from build123d import *

# Parameters (mm, degrees)
SKETCH2_W               = 147.5
SKETCH2_H               = 176.75
BOSS_EXTRUDE1_DEPTH     = 10
SKETCH3_W               = 29
SKETCH3_H               = 15
BOSS_EXTRUDE2_DEPTH     = 34
BOSS_EXTRUDE3_DEPTH     = 34
SKETCH8_W               = 113.5
SKETCH8_H               = 176.75
CUT_EXTRUDE1_DEPTH      = 30
SKETCH9_R               = 2.5
CUT_EXTRUDE2_DEPTH      = 134.016415209
SKETCH10_W              = 3
SKETCH10_H              = 3
CUT_EXTRUDE3_DEPTH      = 3
CUT_EXTRUDE4_DEPTH      = 134.016415209
CUT_EXTRUDE4_DEPTH_BACK = 134.016415209
SKETCH11_W              = 9
SKETCH11_H              = 8
SKETCH11_H_2            = 4
SKETCH11_W_2            = 3
SKETCH11_R              = 2.5
SKETCH11_W_3            = 34
SKETCH11_H_3            = 15
CUT_EXTRUDE5_DEPTH      = 94.691731892
CUT_EXTRUDE5_DEPTH_BACK = 94.691731892
SKETCH13_R              = 2.5
CUT_EXTRUDE6_DEPTH      = 94.691731892
CUT_EXTRUDE6_DEPTH_BACK = 94.691731892
SKETCH14_W              = 10
SKETCH14_H              = 2
FILLET1_R               = 2
SKETCH15_R              = 1.4
CUT_EXTRUDE7_DEPTH      = 34
SKETCH18_W              = 12
SKETCH18_H              = 8
CUT_EXTRUDE8_DEPTH      = 34
SKETCH19_W              = 7
SKETCH19_H              = 8
SKETCH19_W_2            = 12
CUT_EXTRUDE9_DEPTH      = 34
BOSS_EXTRUDE4_START     = 5
SKETCH20_W              = 34
SKETCH20_H              = 29
SKETCH20_R              = 1.4
BOSS_EXTRUDE4_DEPTH     = 5
SKETCH21_W              = 34
SKETCH21_H              = 29
SKETCH21_W_2            = 10
SKETCH21_H_2            = 10
CUT_EXTRUDE10_DEPTH     = 5
SKETCH22_W              = 10
SKETCH22_H              = 3
CUT_EXTRUDE11_DEPTH     = 1


with BuildPart() as part:
    # Sketch2 → Boss-Extrude1 (new body)
    with BuildSketch(Plane.XY):
        Rectangle(SKETCH2_W, SKETCH2_H)
    extrude(amount=BOSS_EXTRUDE1_DEPTH)

    # Sketch3 → Boss-Extrude2 (add)
    with BuildSketch(Plane.ZY.offset(73.75)):
        with Locations((7.5, 80.875)):
            Rectangle(SKETCH3_W, SKETCH3_H)
        with Locations((7.5, -80.875)):
            Rectangle(SKETCH3_W, SKETCH3_H)
    boss_extrude2 = extrude(amount=-BOSS_EXTRUDE2_DEPTH)

    # Mirror1: Boss-Extrude2 across plane
    add(boss_extrude2.mirror(Plane(origin=(0, 0, 0), x_dir=(0, 0, 1), z_dir=(1, 0, 0))))

    # Sketch5 → Boss-Extrude3 (add)
    with BuildSketch(Plane.ZY.offset(73.75)):
        Polygon((13.717233978, 0), (47.494362324, 23.650999887), (54.37727956, 13.821175356), (66.664560225, 22.424821901), (50.030843571, 46.180231185), (37.743562906, 37.57658464), (41.758597961, 31.84252033), (10, 9.604910635), (10, -9.604910635), (41.758597961, -31.84252033), (37.743562906, -37.57658464), (50.030843571, -46.180231185), (66.664560225, -22.424821901), (54.37727956, -13.821175356), (47.494362324, -23.650999887), align=None)
    extrude(amount=-BOSS_EXTRUDE3_DEPTH)

    # Sketch8 → Cut-Extrude1 (cut)
    with BuildSketch(Plane.XY.offset(22)):
        with Locations((17, 0)):
            Rectangle(SKETCH8_W, SKETCH8_H)
    extrude(amount=-CUT_EXTRUDE1_DEPTH, mode=Mode.SUBTRACT)

    # Sketch9 → Cut-Extrude2 (cut, through all)
    with BuildSketch(Plane(origin=(0, 0, 0), x_dir=(-1, 0, 0), z_dir=(0, 0, -1))):
        with Locations((49.75, 58.375)):
            Circle(SKETCH9_R)
        with Locations((63.75, 58.375)):
            Circle(SKETCH9_R)
        with Locations((49.75, -53.375)):
            Circle(SKETCH9_R)
        with Locations((63.75, -53.375)):
            Circle(SKETCH9_R)
    extrude(amount=-CUT_EXTRUDE2_DEPTH, mode=Mode.SUBTRACT)

    # Sketch10 → Cut-Extrude3 (cut)
    with BuildSketch(Plane(origin=(0, 0, -7), x_dir=(-1, 0, 0), z_dir=(0, 0, -1))):
        with Locations((72.25, 86.875)):
            Rectangle(SKETCH10_W, SKETCH10_H)
    extrude(amount=-CUT_EXTRUDE3_DEPTH, mode=Mode.SUBTRACT)

    # Sketch11 → Cut-Extrude4 (cut, two sides: drawn at the far end of the back side and taken through both)
    # profile 1 of 12: a face of its own
    with BuildSketch(Plane(origin=(0, 0, 0), x_dir=(-1, 0, 0), z_dir=(0, 0, -1)).offset(-CUT_EXTRUDE4_DEPTH_BACK)):
        with Locations((47.25, -69.375)):
            Rectangle(SKETCH11_W, SKETCH11_H)
    # profile 2 of 12: a face of its own
    with BuildSketch(Plane(origin=(0, 0, 0), x_dir=(-1, 0, 0), z_dir=(0, 0, -1)).offset(-CUT_EXTRUDE4_DEPTH_BACK)):
        with Locations((47.25, -63.375)):
            Rectangle(SKETCH11_W, SKETCH11_H_2)
    # profile 3 of 12: a face of its own
    with BuildSketch(Plane(origin=(0, 0, 0), x_dir=(-1, 0, 0), z_dir=(0, 0, -1)).offset(-CUT_EXTRUDE4_DEPTH_BACK)):
        with Locations((41.25, -69.375)):
            Rectangle(SKETCH11_W_2, SKETCH11_H)
    # profile 4 of 12: a face of its own
    with BuildSketch(Plane(origin=(0, 0, 0), x_dir=(-1, 0, 0), z_dir=(0, 0, -1)).offset(-CUT_EXTRUDE4_DEPTH_BACK)):
        with Locations((41.25, -63.375)):
            Rectangle(SKETCH11_W_2, SKETCH11_H_2)
    # profile 5 of 12: a face of its own
    with BuildSketch(Plane(origin=(0, 0, 0), x_dir=(-1, 0, 0), z_dir=(0, 0, -1)).offset(-CUT_EXTRUDE4_DEPTH_BACK)):
        with Locations((66.25, -69.375)):
            Rectangle(SKETCH11_W, SKETCH11_H)
    # profile 6 of 12: a face of its own
    with BuildSketch(Plane(origin=(0, 0, 0), x_dir=(-1, 0, 0), z_dir=(0, 0, -1)).offset(-CUT_EXTRUDE4_DEPTH_BACK)):
        with Locations((66.25, -63.375)):
            Rectangle(SKETCH11_W, SKETCH11_H_2)
    # profile 7 of 12: a face of its own
    with BuildSketch(Plane(origin=(0, 0, 0), x_dir=(-1, 0, 0), z_dir=(0, 0, -1)).offset(-CUT_EXTRUDE4_DEPTH_BACK)):
        with Locations((72.25, -63.375)):
            Rectangle(SKETCH11_W_2, SKETCH11_H_2)
    # profile 8 of 12: a face of its own
    with BuildSketch(Plane(origin=(0, 0, 0), x_dir=(-1, 0, 0), z_dir=(0, 0, -1)).offset(-CUT_EXTRUDE4_DEPTH_BACK)):
        with Locations((72.25, -69.375)):
            Rectangle(SKETCH11_W_2, SKETCH11_H)
    # profile 9 of 12: a face of its own
    with BuildSketch(Plane(origin=(0, 0, 0), x_dir=(-1, 0, 0), z_dir=(0, 0, -1)).offset(-CUT_EXTRUDE4_DEPTH_BACK)):
        Polygon((39.75, 73.375), (39.75, -58.375), (51.75, -58.375), (61.75, -58.375), (73.75, -58.375), (73.75, 73.375), align=None)
        with Locations((49.75, -53.375)):
            Circle(SKETCH11_R, mode=Mode.SUBTRACT)
        with Locations((63.75, -53.375)):
            Circle(SKETCH11_R, mode=Mode.SUBTRACT)
        with Locations((49.75, 58.375)):
            Circle(SKETCH11_R, mode=Mode.SUBTRACT)
        with Locations((63.75, 58.375)):
            Circle(SKETCH11_R, mode=Mode.SUBTRACT)
    # profile 10 of 12: a face of its own
    with BuildSketch(Plane(origin=(0, 0, 0), x_dir=(-1, 0, 0), z_dir=(0, 0, -1)).offset(-CUT_EXTRUDE4_DEPTH_BACK)):
        Polygon((61.75, -58.375), (61.75, -61.375), (70.75, -61.375), (73.75, -61.375), (73.75, -58.375), align=None)
    # profile 11 of 12: a face of its own
    with BuildSketch(Plane(origin=(0, 0, 0), x_dir=(-1, 0, 0), z_dir=(0, 0, -1)).offset(-CUT_EXTRUDE4_DEPTH_BACK)):
        Polygon((39.75, -58.375), (39.75, -61.375), (42.75, -61.375), (51.75, -61.375), (51.75, -58.375), align=None)
    # profile 12 of 12: a face of its own
    with BuildSketch(Plane(origin=(0, 0, 0), x_dir=(-1, 0, 0), z_dir=(0, 0, -1)).offset(-CUT_EXTRUDE4_DEPTH_BACK)):
        with Locations((56.75, 80.875)):
            Rectangle(SKETCH11_W_3, SKETCH11_H_3)
    extrude(amount=CUT_EXTRUDE4_DEPTH + CUT_EXTRUDE4_DEPTH_BACK, mode=Mode.SUBTRACT)

    # Sketch13 → Cut-Extrude5 (cut, two sides: drawn at the far end of the back side and taken through both)
    with BuildSketch(Plane.ZY.offset(61.75).offset(-CUT_EXTRUDE5_DEPTH_BACK)):
        with Locations((5, -63.375)):
            Circle(SKETCH13_R)
    extrude(amount=CUT_EXTRUDE5_DEPTH + CUT_EXTRUDE5_DEPTH_BACK, mode=Mode.SUBTRACT)

    # Sketch14 → Cut-Extrude6 (cut, two sides: drawn at the far end of the back side and taken through both)
    with BuildSketch(Plane.ZY.offset(61.75).offset(-CUT_EXTRUDE6_DEPTH_BACK)):
        with Locations((5, -59.375)):
            Rectangle(SKETCH14_W, SKETCH14_H)
    extrude(amount=CUT_EXTRUDE6_DEPTH + CUT_EXTRUDE6_DEPTH_BACK, mode=Mode.SUBTRACT)

    # Fillet1
    fillet1_edges = [part.edges().sort_by_distance(p)[0] for p in [
        (-56.75, -60.375, 0),
        (-56.75, -60.375, 10),
    ]]
    fillet(fillet1_edges, radius=FILLET1_R)

    # Sketch15 → Cut-Extrude7 (cut)
    with BuildSketch(Plane.XZ.offset(88.375)):
        with Locations(Location((-46.75, -1.8, 0), (0, 0, 270))):
            Circle(SKETCH15_R)
        with Locations(Location((-66.75, -1.8, 0), (0, 0, 270))):
            Circle(SKETCH15_R)
        with Locations(Location((-66.75, 14.2, 0), (0, 0, 270))):
            Circle(SKETCH15_R)
        with Locations(Location((-46.75, 14.2, 0), (0, 0, 270))):
            Circle(SKETCH15_R)
    extrude(amount=-CUT_EXTRUDE7_DEPTH, mode=Mode.SUBTRACT)

    # Sketch18 → Cut-Extrude8 (cut)
    with BuildSketch(Plane(origin=(0, 0, -7), x_dir=(-1, 0, 0), z_dir=(0, 0, -1))):
        with Locations((45.75, -77.375)):
            Rectangle(SKETCH18_W, SKETCH18_H)
        with Locations((67.75, -77.375)):
            Rectangle(SKETCH18_W, SKETCH18_H)
    extrude(amount=-CUT_EXTRUDE8_DEPTH, mode=Mode.SUBTRACT)

    # Sketch19 → Cut-Extrude9 (cut)
    with BuildSketch(Plane.ZY.offset(61.75)):
        with Locations((-3.5, -77.375)):
            Rectangle(SKETCH19_W, SKETCH19_H)
        with Locations((16, -77.375)):
            Rectangle(SKETCH19_W_2, SKETCH19_H)
    extrude(amount=-CUT_EXTRUDE9_DEPTH, mode=Mode.SUBTRACT)

    # Sketch20 → Boss-Extrude4 (add)
    with BuildSketch(Plane.XZ.offset(88.375).offset(BOSS_EXTRUDE4_START)):
        with Locations((-56.75, 7.5)):
            Rectangle(SKETCH20_W, SKETCH20_H)
        with Locations(Location((-66.75, 14.2, 0), (0, 0, 270))):
            Circle(SKETCH20_R, mode=Mode.SUBTRACT)
        with Locations(Location((-46.75, 14.2, 0), (0, 0, 270))):
            Circle(SKETCH20_R, mode=Mode.SUBTRACT)
        with Locations(Location((-46.75, -1.8, 0), (0, 0, 270))):
            Circle(SKETCH20_R, mode=Mode.SUBTRACT)
        with Locations(Location((-66.75, -1.8, 0), (0, 0, 270))):
            Circle(SKETCH20_R, mode=Mode.SUBTRACT)
    extrude(amount=-BOSS_EXTRUDE4_DEPTH)

    # Sketch21 → Cut-Extrude10 (cut)
    with BuildSketch(Plane(origin=(0, -81.375, 0), x_dir=(1, 0, 0), z_dir=(0, 1, 0))):
        with Locations((-56.75, -7.5)):
            Rectangle(SKETCH21_W, SKETCH21_H)
        with Locations((-56.75, -5)):
            Rectangle(SKETCH21_W_2, SKETCH21_H_2, mode=Mode.SUBTRACT)
    extrude(amount=-CUT_EXTRUDE10_DEPTH, mode=Mode.SUBTRACT)

    # Sketch22 → Cut-Extrude11 (cut)
    with BuildSketch(Plane.XY.offset(10)):
        with Locations((-56.75, -72.875)):
            Rectangle(SKETCH22_W, SKETCH22_H)
    extrude(amount=-CUT_EXTRUDE11_DEPTH, mode=Mode.SUBTRACT)


solid = part.part
Could you check a few things on this model? Use its own coordinates, in mm. A direction names the side the tool comes from. Give positions to 0.01 mm unless a question says otherwise; leave off trailing zeros. Loops run counter-clockwise (first coordinate to the right, second up) from the corner with the lowest first, then second, coordinate; pieces in that order, holes last. Notation, with made-up numbers: M -39,-5.75 L -34,-5.75 A29 ccw -34,19.25 Z; hole C 3,-2.75 d7. An arc over 180 degrees is marked long. Answer as a JSON object with one key per item and string values.
Q1. If I drill on probe 1 along X at (y, z) = (-90.25, -1.8); probe 2 along Z at (x, y) = (-66.75, -89); probe 3 along Y at (x, z) = (-58.75, 5) (3 decimals), over which ranges is the centre line in solid material (lowest first)? Write a range as [from, to].
Values found:
{"probe 1": "x = [-73.75, -68.15], [-65.35, -48.15], [-45.35, -39.75]", "probe 2": "z = [-7, -3.2], [-0.4, 12.8], [15.6, 22]", "probe 3": "y = [-93.375, -65.875], [-60.875, -60.375]"}
Q2. Suppose I cut it at D-D, the plane z = 5. List the corners of the cut face in (x, y) for me (3 decimals), plus the area to 3 significant figures.
Values found:
{"outline": "M -73.75,-93.375 L -39.75,-93.375 L -39.75,-86.375 L -51.75,-86.375 L -51.75,-65.875 L -61.75,-65.875 L -61.75,-86.375 L -73.75,-86.375 Z; M -61.75,-60.875 L -51.75,-60.875 L -51.75,-60.375 L -61.75,-60.375 Z", "area": "448 mm²"}
Q3. Suppose I cut it at C-C, the plane x = -46.75. List the corners of the cut face in (y, z) for me (3 decimals), plus the area to 3 significant figures.
Values found:
{"outline": "M -93.375,-7 L -86.375,-7 L -86.375,-3.2 L -93.375,-3.2 Z; M -93.375,-0.4 L -86.375,-0.4 L -86.375,12.8 L -93.375,12.8 Z; M -93.375,15.6 L -86.375,15.6 L -86.375,22 L -93.375,22 Z", "area": "164 mm²"}
Q4. Suppose I cut it at A-A, the plane y = -90.5. List the corners of the cut face in (x, z) for me, plus the area to 3 significant figures.
Values found:
{"outline": "M -73.75,-7 L -39.75,-7 L -39.75,22 L -73.75,22 Z; hole C -66.75,-1.8 d2.8; hole C -66.75,14.2 d2.8; hole C -46.75,-1.8 d2.8; hole C -46.75,14.2 d2.8", "area": "961 mm²"}
Q5. For P1, Ø3, axis at x = -52.5, y = -69, coming from the +Z side; P2, Ø5, axis at y = -73, z = 6.5, coming from the +X side; P3, Ø8, axis at x = -65.5, y = -69, coming from the -Z side, each with a flat end and sliding along its axis, tell me the tip position at first contact or that it passes through.
Values found:
{"P1": "stops at z = 10", "P2": "stops at x = -51.75", "P3": "stops at z = 0"}
Q6. Suppose I cut it at B-B, the plane z = 14.2. List the corners of the cut face in (x, y) for me (3 decimals).
Values found:
{"outline": "M -73.75,-93.375 L -68.15,-93.375 L -68.15,-86.375 L -73.75,-86.375 Z; M -65.35,-93.375 L -48.15,-93.375 L -48.15,-86.375 L -65.35,-86.375 Z; M -45.35,-93.375 L -39.75,-93.375 L -39.75,-86.375 L -45.35,-86.375 Z"}
Q7. If we mould it in two halves opening along X, with no side actions, what happens to faces 4 (the flat face through (-39.75, -90, 7)), 5 (the flat face through (-57, -90, 22)), 6 (the flat face through (-61.75, -73, 5)), 7 (the cylindrical face through (-45.36, -89.92, -1.62))? For each: pulls with the +X half, pulls with the -X half, needs draft (parallel to the pull), parting line crosses it, or undercut.
Values found:
{"face 4": "pulls with the +X half", "face 5": "needs draft", "face 6": "pulls with the -X half", "face 7": "undercut"}
Q8. For faces 1 (the flat face through (-51.75, -73, 5)), 2 (the flat face through (-56.8, -74.375, 9.5)), 3 (the flat face through (-57, -74, 0)), which set-ups out of +Z, -Z, +X, -X, +Y, -Y let a thin tool reach every point of the face, with its end or its side?
Values found:
{"face 1": "+Z, -Z, +X, +Y", "face 2": "+Z, +X, -X", "face 3": "-Z, +X, -X, +Y"}
